Could you check a few things on this model? Use its own coordinates, in mm. Round coordinates to 2 decimals unless told otherwise and drop trailing zeros. Loops run counter-clockwise (first coordinate to the right, second up) from the corner with the lowest first, then second, coordinate; pieces in that order, holes last. Notation, with made-up numbers: (88.25, -9) - (95.25, -9) arc R26 cw to (95.25, 22) - close; hole circle Ø11 at (36, 27). An arc over 180 degrees is marked (long way). Answer as CSV lines item,"result". Start each with the question number.
1) Suppose I cut it at B-B, the plane x = -65. Write out the boundary of the cut face in (y, z).
2) Suppose I cut it at C-C, the plane z = -75.5. Write out the boundary of the cut face in (x, y).
3) I'm going to push flat-ended pins straight in: pin 1 Ø3 at (x, z) = (65, 37.5) entering from -Y; pin 2 Ø6 at (x, y) = (-39.5, 3.5) entering from -Z; pin 3 Ø6 at (x, y) = (-23.5, 8) entering from -Z; pin 4 Ø3 at (x, y) = (26.5, 8) entering from +Z. Where does each tip first touch, or does it pass through?
4) Suppose I cut it at D-D, the plane y = 8. Count the separate pieces of the cut face and the enclosed holes in it, then the cut area to 3 significant figures.
5) Please list where these lines run through material, in increasing order: line 1 along Z through (x, y) = (0, 6.5); line 2 along X through (y, z) = (8.5, -37.5); line 3 along Z through (x, y) = (-36, 7.25).
6) Suppose I cut it at A-A, the plane z = 37.5. Write out the boundary of the cut face in (x, y).
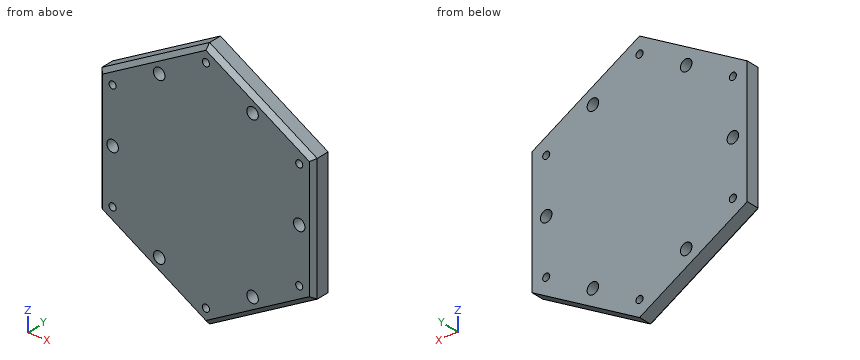
```python
from build123d import *

# Parameters (mm, degrees)
EXTRUDE_1_DEPTH     = 12
CHAMFER_1_SIZE      = 3
SKETCH_2_R          = 4
EXTRUDE_2_DEPTH     = 12
HOLE_WIZARD_1_D     = 4.917
HOLE_WIZARD_1_DEPTH = 17.1
HOLE_WIZARD_1_TIP   = 1.477215832


with BuildPart() as part:
    # 草圖1 → 擠出1 (new body)
    with BuildSketch(Plane(origin=(0, 0, 0), x_dir=(-1, 0, 0), z_dir=(0, 1, 0))):
        Polygon((0, -86.602540378), (-75, -43.301270189), (-75, 43.301270189), (0, 86.602540378), (75, 43.301270189), (75, -43.301270189), align=None)
    extrude(amount=EXTRUDE_1_DEPTH)

    # 倒角1
    chamfer_1_edges = [part.edges().sort_by_distance(p)[0] for p in [
        (37.5, 0, -64.951905284),
        (75, 0, 0),
        (37.5, 0, 64.951905284),
        (-37.5, 0, 64.951905284),
        (-75, 0, 0),
        (-37.5, 0, -64.951905284),
    ]]
    chamfer(chamfer_1_edges, length=CHAMFER_1_SIZE)

    # 草圖2 → 擠出2 (cut)
    with BuildSketch(Plane(origin=(0, 12, 0), x_dir=(-1, 0, 0), z_dir=(0, 1, 0))):
        with Locations(Location((-32.5, 56.5, 0), (0, 0, 90))):
            Circle(SKETCH_2_R)
        with Locations(Location((32.5, 56.5, 0), (0, 0, 90))):
            Circle(SKETCH_2_R)
        with Locations(Location((-65, 0, 0), (0, 0, 90))):
            Circle(SKETCH_2_R)
        with Locations(Location((-32.5, -56.5, 0), (0, 0, 90))):
            Circle(SKETCH_2_R)
        with Locations(Location((32.5, -56.5, 0), (0, 0, 90))):
            Circle(SKETCH_2_R)
        with Locations(Location((65, 0, 0), (0, 0, 90))):
            Circle(SKETCH_2_R)
    extrude(amount=-EXTRUDE_2_DEPTH, mode=Mode.SUBTRACT)

    # 孔1
    with Locations(Plane(origin=(0, 12, 0), x_dir=(1, 0, 0), z_dir=(0, 1, 0))):
        with Locations((0, 75.5), (-65, 37.5), (65, 37.5), (-65, -37.5), (65, -37.5), (0, -75.5)):
            Hole(HOLE_WIZARD_1_D / 2, depth=HOLE_WIZARD_1_DEPTH)
            with Locations((0, 0, -(HOLE_WIZARD_1_DEPTH + HOLE_WIZARD_1_TIP / 2))):  # 118° drill point
                Cone(0, HOLE_WIZARD_1_D / 2, HOLE_WIZARD_1_TIP, mode=Mode.SUBTRACT)


solid = part.part
```
Filled sheet:
1,outline,"(0, -45.61) - (3, -49.07) - (12, -49.07) - (12, -39.96) - (0, -39.96) - close; (0, -35.04) - (12, -35.04) - (12, -4) - (0, -4) - close; (0, 4) - (12, 4) - (12, 35.04) - (0, 35.04) - close; (0, 39.96) - (12, 39.96) - (12, 49.07) - (3, 49.07) - (0, 45.61) - close"
2,outline,"(-19.23, 3) - (-13.23, 0) - (-2.46, 0) - (-2.46, 12) - (-19.23, 12) - close; (2.46, 0) - (13.23, 0) - (19.23, 3) - (19.23, 12) - (2.46, 12) - close"
3,pin 1,"through"
3,pin 2,"z = -65.53"
3,pin 3,"z = -74.77"
3,pin 4,"z = 72.17"
4,separate pieces,"1"
4,enclosed holes,"12"
4,area,"19,100 mm²"
5,line 1,"-86.6 to -77.96, -73.04 to 73.04, 77.96 to 86.6"
5,line 2,"-75 to -67.46, -62.54 to 62.54, 67.46 to 75"
5,line 3,"-65.82 to -58.44, -54.56 to 54.56, 58.44 to 65.82"
6,outline,"(-75, 3) - (-72, 0) - (-67.46, 0) - (-67.46, 12) - (-75, 12) - close; (-62.54, 0) - (62.54, 0) - (62.54, 12) - (-62.54, 12) - close; (67.46, 0) - (72, 0) - (75, 3) - (75, 12) - (67.46, 12) - close"
